Check sheet for the drawn part. Datum: minimum x, y, z corner. Units: mm. A direction names the side the tool comes from. Give positions to 0.01 mm unless a question says otherwise; leave off trailing zeros. Order: outer loops, then holes, each group sorted by start corner. A loop starts at its lowest first (then second) coordinate and runs counter-clockwise, first axis right, second up. Notation, with made-up numbers: (55, 5) -> (66, 5) arc R28 cw to (66, 25) -> close; hole circle Ø11 at (-0.5, -10). An arc over 180 degrees is marked (long way). One line per question, with ' | ' between items. Start each with the question number.
Q1. Go/stop test with flat-tipped pins: pin 1 (6 mm diameter, centred on x = 15, y = 2.5, fed in from +Z); pin 2 (3 mm diameter, centred on x = 14, z = 11.5, fed in from -Y); pin 3 (6 mm diameter, centred on x = 9.5, y = 6, fed in from +Z). Record where each tip stops, or that it passes through.
Q2. Material ranges on probe 1 along X at (y, z) = (2.5, 27.2); probe 2 along Z at (x, y) = (4, 13); probe 3 along Y at (x, z) = (2, 5), recorded low to high. Write a range as [from, to].
Q3. Section check D-D on y = 34.5. Record the cut outline in (x, z), plus the area to 3 significant figures.
Q4. Section check B-B on x = 5.5. Record the cut outline in (y, z), plus the area to 3 significant figures.
Q5. Access from +Z, -Z, +X, -X, +Y, -Y to the whole of each face (thin tool, end or side, straight path). Record for the marked faces 1, 2, 3 and 4.
Q6. Section check C-C on x = 10. Record the cut outline in (y, z).
Q7. Section check A-A on y = 52. Record the cut outline in (x, z).
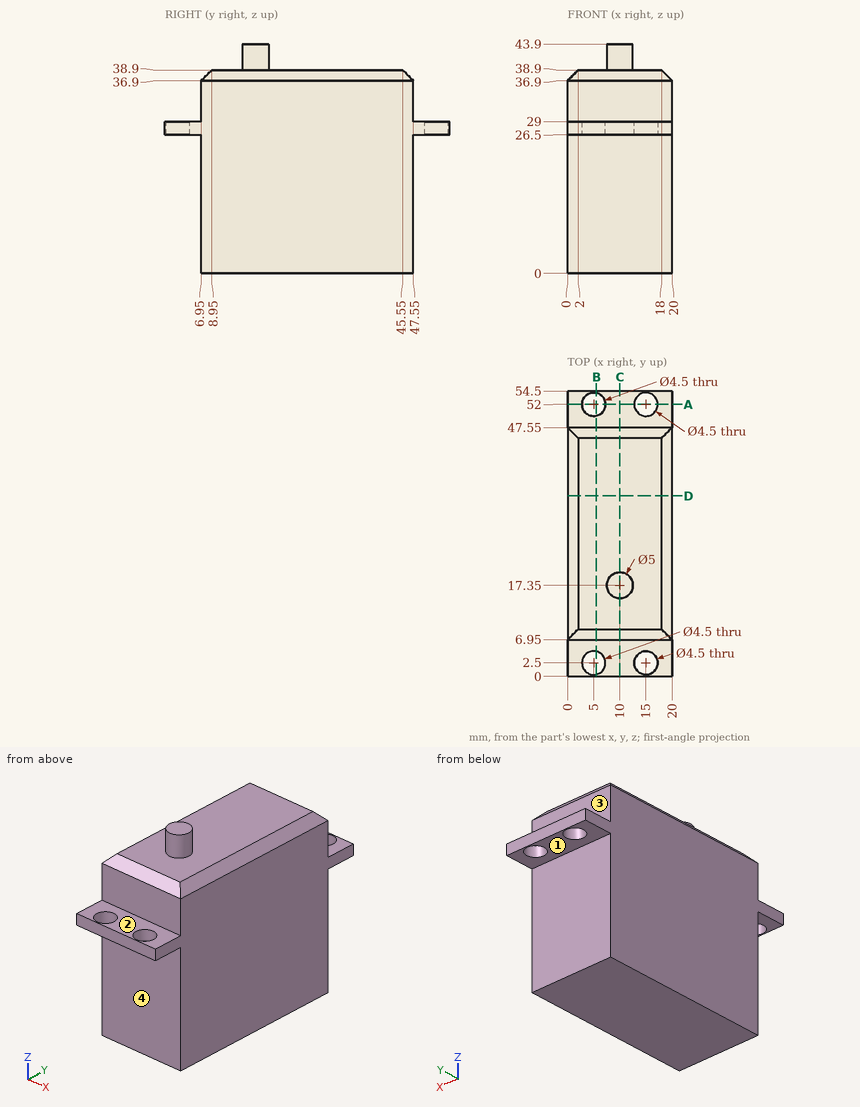
Filled in:
1) pin 1: z = 29 | pin 2: y = 6.95 | pin 3: z = 38.9
2) probe 1: [0, 2.75], [7.25, 12.75], [17.25, 20] | probe 2: [0, 38.9] | probe 3: [6.95, 47.55]
3) outline: (0, 0) -> (20, 0) -> (20, 36.9) -> (18, 38.9) -> (2, 38.9) -> (0, 36.9) -> close | area: 774 mm²
4) outline: (0, 26.5) -> (0.31, 26.5) -> (0.31, 29) -> (0, 29) -> close; (4.69, 26.5) -> (6.95, 26.5) -> (6.95, 0) -> (47.55, 0) -> (47.55, 26.5) -> (49.81, 26.5) -> (49.81, 29) -> (47.55, 29) -> (47.55, 36.9) -> (45.55, 38.9) -> (8.95, 38.9) -> (6.95, 36.9) -> (6.95, 29) -> (4.69, 29) -> close; (54.19, 26.5) -> (54.5, 26.5) -> (54.5, 29) -> (54.19, 29) -> close | area: 1,590 mm²
5) face 1: -Z, +X, -X, +Y | face 2: +Z, +X, -X, -Y | face 3: +Z, +X, -X, +Y | face 4: -Z, +X, -X, -Y
6) outline: (0, 26.5) -> (6.95, 26.5) -> (6.95, 0) -> (47.55, 0) -> (47.55, 26.5) -> (54.5, 26.5) -> (54.5, 29) -> (47.55, 29) -> (47.55, 36.9) -> (45.55, 38.9) -> (19.85, 38.9) -> (19.85, 43.9) -> (14.85, 43.9) -> (14.85, 38.9) -> (8.95, 38.9) -> (6.95, 36.9) -> (6.95, 29) -> (0, 29) -> close
7) outline: (0, 26.5) -> (2.75, 26.5) -> (2.75, 29) -> (0, 29) -> close; (7.25, 26.5) -> (12.75, 26.5) -> (12.75, 29) -> (7.25, 29) -> close; (17.25, 26.5) -> (20, 26.5) -> (20, 29) -> (17.25, 29) -> close
